from build123d import *

# Parameters (mm, degrees)
F0_R     = 1.6
F1_DEPTH = 10
F2_R     = 2
F3_SIZE  = 1


with BuildPart() as f1:
    # F0 (on Top) → F1 (new body)
    with BuildSketch(Plane.XY):
        with BuildLine():
            ThreePointArc((22.309715, 4.280196), (19.411123, 5.989188), (16.840064, 8.159936))
            Line((16.840064, 8.159936), (8.159936, 16.840064))
            ThreePointArc((8.159936, 16.840064), (5.989188, 19.411123), (4.280196, 22.309715))
            ThreePointArc((4.280196, 22.309715), (2.527732, 24.271576), (0, 25))
            ThreePointArc((0, 25), (-2.527732, 24.271576), (-4.280196, 22.309715))
            ThreePointArc((-4.280196, 22.309715), (-5.989188, 19.411123), (-8.159936, 16.840064))
            Line((-8.159936, 16.840064), (-16.840064, 8.159936))
            ThreePointArc((-16.840064, 8.159936), (-19.411123, 5.989188), (-22.309715, 4.280196))
            ThreePointArc((-22.309715, 4.280196), (-24.326044, -2.438928), (-17.45191, -3.838384))
            ThreePointArc((-17.45191, -3.838384), (-13.581355, -1.631059), (-9.318154, -0.335452))
            ThreePointArc((-9.318154, -0.335452), (-5.198131, 0.899152), (-1.437341, 2.986088))
            Line((-1.437341, 2.986088), (-0.576424, 3.593386))
            ThreePointArc((-0.576424, 3.593386), (-0.302365, 3.729427), (0, 3.776235))
            ThreePointArc((0, 3.776235), (0.302365, 3.729427), (0.576424, 3.593386))
            Line((0.576424, 3.593386), (1.437341, 2.986088))
            ThreePointArc((1.437341, 2.986088), (5.198131, 0.899152), (9.318154, -0.335452))
            ThreePointArc((9.318154, -0.335452), (13.581355, -1.631059), (17.45191, -3.838384))
            ThreePointArc((17.45191, -3.838384), (24.326044, -2.438928), (22.309715, 4.280196))
        make_face()
        with Locations((-20.25, 0)):
            Circle(F0_R, mode=Mode.SUBTRACT)
        with Locations((20.25, 0)):
            Circle(F0_R, mode=Mode.SUBTRACT)
        with BuildLine():
            ThreePointArc((0, 21.85), (1.6, 20.25), (0, 18.65))
            ThreePointArc((0, 18.65), (-1.6, 20.25), (0, 21.85))
        make_face(mode=Mode.SUBTRACT)
    extrude(amount=F1_DEPTH)

    # F2
    f2_edges = [f1.edges().sort_by_distance(p)[0] for p in [
        (-5.198131, 0.899152, 10),
        (-5.198131, 0.899152, 0),
        (-12.5, 12.5, 10),
        (-19.411123, 5.989188, 10),
    ]]
    fillet(f2_edges, radius=F2_R)

    # F3
    f3_edges = [f1.edges().sort_by_distance(p)[0] for p in [
        (0, 18.65, 10),
        (-21.85, 0, 10),
        (18.65, 0, 10),
        (-21.85, 0, 0),
        (0, 18.65, 0),
        (18.65, 0, 0),
    ]]
    chamfer(f3_edges, length=F3_SIZE)


solid = f1.part
Here's how the part is built. I have some questions about the finished solid (model axes, mm). A direction names the side the tool comes from. Round coordinates to 2 decimals unless told otherwise and drop trailing zeros. Order: outer loops, then holes, each group sorted by start corner. A loop starts at its lowest first (then second) coordinate and runs counter-clockwise, first axis right, second up. Notation, with made-up numbers: M 89.5,47 L 143.5,47 A35 ccw 143.5,85 Z; hole C -22.5,16 d5. An arc over 180 degrees is marked long. One line per question, with ' | ' between items.
1) On a 3-axis mill with a long thin cutter (end or side, diameter ignored), from which of +Z, -Z, +X, -X, +Y, -Y can I reach the whole of each face in a straight line? I mean faces 5 (the cylindrical face through (1.342, 3.752, 0.601)), 6 (the cylindrical face through (-5.96, 19.45, 4.96)), 7 (the cylindrical face through (1.342, 3.752, 9.399)). Say none if no direction works.
Checked values:
face 5: -Z, -Y | face 6: +Z, -Z, -X, +Y | face 7: +Z, -Y
2) Imagine slicing it at B-B, the plane y = -1. Count the separate pieces of the cut face and the enclosed holes in it, plus the area to 3 significant figures.
Checked values:
separate pieces: 4 | enclosed holes: 0 | area: 192 mm²
3) Imagine slicing it at A-A, the plane z = 3.5. Write out the boundary of the cut face in (x, y), plus the area to 3 significant figures.
Checked values:
outline: M -22.31,4.28 A4.75 ccw long -17.45,-3.84 A20 cw -9.32,-0.34 A20 ccw -1.44,2.99 L -0.58,3.59 A1 cw 0,3.78 A1 cw 0.58,3.59 L 1.44,2.99 A20 ccw 9.32,-0.34 A20 cw 17.45,-3.84 A4.75 ccw long 22.31,4.28 A20 cw 16.84,8.16 L 8.16,16.84 A20 cw 4.28,22.31 A4.75 ccw 0,25 A4.75 ccw -4.28,22.31 A20 cw -8.16,16.84 L -16.84,8.16 A20 cw Z; hole C -20.25,0 d3.2; hole C 0,20.25 d3.2; hole C 20.25,0 d3.2 | area: 695 mm²
4) I need wall thicknesses on line 1 (Y direction, x = 20.25, z = 7.25); line 2 (X direction, y = 20.25, z = 3); line 3 (Y direction, x = -21, z = 6). Which ranges of each line are inside material? Lowest first, please.
Checked values:
line 1: y = -4.75 to -1.6, 1.6 to 5.43 | line 2: x = -5.43 to -1.6, 1.6 to 5.43 | line 3: y = -4.69 to -1.41, 1.41 to 4.97
5) Imagine slicing it at C-C, the plane z = 8.5. Write out the boundary of the cut face in (x, y), plus the area to 3 significant figures.
Checked values:
outline: M -22.28,4.22 A4.69 ccw long -17.49,-3.79 A20.06 cw -9.33,-0.27 A19.94 ccw -1.47,3.04 L -0.61,3.65 A1.06 cw 0,3.84 A1.06 cw 0.61,3.65 L 1.47,3.04 A19.94 ccw 9.33,-0.27 A20.06 cw 17.49,-3.79 A4.69 ccw long 22.28,4.22 A20.06 cw 16.8,8.12 L 8.12,16.8 A20.06 cw 4.22,22.28 A4.69 ccw 0,24.94 A4.69 ccw -4.22,22.28 A20.06 cw -8.12,16.8 L -16.8,8.12 A20.06 cw Z; hole C -20.25,0 d3.2; hole C 0,20.25 d3.2; hole C 20.25,0 d3.2 | area: 686 mm²
6) I'm going to push flat-ended pins straight in: pin 1 Ø1.5 at (y, z) = (16, 2) entering from +X; pin 2 Ø3 at (x, z) = (-2.5, 3) entering from +Y; pin 3 Ø5 at (x, y) = (20.25, 0) entering from -Z. Where does each tip first touch, or does it pass through?
Checked values:
pin 1: stops at x = 9.75 | pin 2: stops at y = 24.89 | pin 3: stops at z = 0.1
7) We'd pull the mould along Y, two halves only. Please class faces 1 (the cylindrical face through (24.27, -2.53, 4.96)), 2 (the cylindrical face through (13.524, -1.606, 4.958)), 3 (the cylindrical face through (19.45, 5.96, 4.96)), 4 (the cylindrical face through (-0.07, 21.85, 4.94)): released by +Y, released by -Y, zero draft, split by the parting line, or undercut.
Checked values:
face 1: split by the parting line | face 2: released by -Y | face 3: released by +Y | face 4: undercut
